Can you work these out from the model? Positions are in its coordinate system, mm. A direction names the side the tool comes from. Round coordinates to 2 decimals unless told otherwise and drop trailing zeros. Write each loop counter-clockwise with the first axis right and the second up, starting at its lowest first coordinate (ties: lowest second). Pieces come first, ordered by that corner, then holes. Notation, with made-up numbers: (13.5, -35) - (35.5, -35) arc R14 cw to (35.5, -19) - close; hole circle Ø4 at (13, 39). An arc over 180 degrees is marked (long way). One line per item, written item: value. Start each with the question number.
(1) I want a section at A-A on z = -2.75. List the corners of the cut face in (x, y) for me.
(2) If I drill on L1, parallel to X at y = 1.3, z = -6; L2, parallel to X at y = 2.2, z = -1.75; L3, parallel to Z at x = 5.5, y = 2.15, over which ranges is the centre line in solid material (lowest first)? Write a range as from..to.
(3) I want a section at D-D on z = 4.75. List the corners of the cut face in (x, y) for me.
(4) I'm going to push flat-ended pins straight in: pin 1 Ø6 at (x, z) = (-21.5, -2.5) entering from -Y; pin 2 Ø1 at (x, y) = (22, 2) entering from -Z; pin 3 Ø0.7 at (x, y) = (2.5, 2) entering from +Z; pin 4 Ø1 at (y, z) = (2, -1) entering from -X. Where does each tip first touch, or does it pass through?
(5) I want a section at C-C on y = 1.05. List the corners of the cut face in (x, z) for me, plus the area to 3 significant figures.
(6) On a 3-axis mill with a long thin cutter (end or side, diameter ignored), from which of +Z, -Z, +X, -X, +Y, -Y can I reach the whole of each face in a straight line? I mean faces 4 (the face through (25.49, 1.89, -5.55)), 5 (the face through (10.699, 0.715, -7.715)), 6 (the face through (0, 2, -6.45)), 7 (the face through (26.35, 2, 0)). Say none if no direction works.
(7) I want a section at B-B on x = -5.5. List the corners of the cut face in (y, z) for me, plus the area to 3 significant figures.
(8) Thinking about a two-plate mould opening in X: for faces 1 (the face through (-28.25, 1, 0)), 2 (the face through (-19, 1, -3)), 3 (the face through (28.25, 1, 0)), which applies, +X half, -X half, draft (parallel to the pull), parting line (faces both ways), or undercut?
from build123d import *

# Parameters (mm, degrees)
BOSS_EXTRUDE1_DEPTH = 1.45
BOSS_EXTRUDE2_DEPTH = 0.9
CUT_EXTRUDE1_DEPTH  = 30.454795874
FILLET1_R           = 1


with BuildPart() as part:
    # Sketch1 → Boss-Extrude1 (new body)
    with BuildSketch(Plane(origin=(0, 0, 0), x_dir=(1, 0, 0), z_dir=(0, 1, 0))):
        with BuildLine():
            Line((-26.25, -8), (26.25, -8))
            ThreePointArc((26.25, -8), (27.664213562, -7.414213562), (28.25, -6))
            Line((28.25, -6), (28.25, 6))
            ThreePointArc((28.25, 6), (27.664213562, 7.414213562), (26.25, 8))
            Line((26.25, 8), (-26.25, 8))
            ThreePointArc((-26.25, 8), (-27.664213562, 7.414213562), (-28.25, 6))
            Line((-28.25, 6), (-28.25, -6))
            ThreePointArc((-28.25, -6), (-27.664213562, -7.414213562), (-26.25, -8))
        make_face()
    extrude(amount=BOSS_EXTRUDE1_DEPTH)

    # Sketch2 → Boss-Extrude2 (add)
    with BuildSketch(Plane(origin=(0, 1.45, 0), x_dir=(1, 0, 0), z_dir=(0, 1, 0))):
        with BuildLine():
            Line((-23.35, -6.45), (23.35, -6.45))
            ThreePointArc((23.35, -6.45), (25.471320344, -5.571320344), (26.35, -3.45))
            Line((26.35, -3.45), (26.35, 3.45))
            ThreePointArc((26.35, 3.45), (25.471320344, 5.571320344), (23.35, 6.45))
            Line((23.35, 6.45), (-23.35, 6.45))
            ThreePointArc((-23.35, 6.45), (-25.471320344, 5.571320344), (-26.35, 3.45))
            Line((-26.35, 3.45), (-26.35, -3.45))
            ThreePointArc((-26.35, -3.45), (-25.471320344, -5.571320344), (-23.35, -6.45))
        make_face()
    extrude(amount=BOSS_EXTRUDE2_DEPTH)

    # Sketch3 → Cut-Extrude1 (cut, through all)
    with BuildSketch(Plane(origin=(0, 2.35, 0), x_dir=(1, 0, 0), z_dir=(0, 1, 0))):
        with BuildLine():
            Line((-19, 0), (-19, 8))
            Line((-19, 8), (-11, 8))
            Line((-11, 8), (-11, 0))
            ThreePointArc((-11, 0), (-15, -4), (-19, 0))
        make_face()
        with BuildLine():
            Line((11, 0), (11, 8))
            Line((11, 8), (19, 8))
            Line((19, 8), (19, 0))
            ThreePointArc((19, 0), (15, -4), (11, 0))
        make_face()
    extrude(amount=-CUT_EXTRUDE1_DEPTH, mode=Mode.SUBTRACT)

    # Fillet1
    fillet1_edges = [part.edges().sort_by_distance(p)[0] for p in [
        (11, 0.725, -8),
        (19, 0.725, -8),
        (-19, 0.725, -8),
        (-11, 0.725, -8),
    ]]
    fillet(fillet1_edges, radius=FILLET1_R)


solid = part.part
Established:
1. outline: (-28.25, 0) - (-19, 0) - (-19, 2.35) - (-26.35, 2.35) - (-26.35, 1.45) - (-28.25, 1.45) - close; (-11, 0) - (11, 0) - (11, 2.35) - (-11, 2.35) - close; (19, 0) - (28.25, 0) - (28.25, 1.45) - (26.35, 1.45) - (26.35, 2.35) - (19, 2.35) - close
2. L1: -28.25..-19, -11..11, 19..28.25
2. L2: -26.35..-19, -11..11, 19..26.35
2. L3: -6.45..6.45
3. outline: (-28.25, 0) - (28.25, 0) - (28.25, 1.45) - (26.05, 1.45) - (26.05, 2.35) - (-26.05, 2.35) - (-26.05, 1.45) - (-28.25, 1.45) - close
4. pin 1: y = 0
4. pin 2: z = -6.45
4. pin 3: z = 6.45
4. pin 4: x = -26.35
5. outline: (-28.25, -6) arc R2 ccw to (-26.25, -8) - (-20, -8) arc R1 ccw to (-19, -7) - (-19, 0) arc R4 cw to (-11, 0) - (-11, -7) arc R1 ccw to (-10, -8) - (10, -8) arc R1 ccw to (11, -7) - (11, 0) arc R4 cw to (19, 0) - (19, -7) arc R1 ccw to (20, -8) - (26.25, -8) arc R2 ccw to (28.25, -6) - (28.25, 6) arc R2 ccw to (26.25, 8) - (-26.25, 8) arc R2 ccw to (-28.25, 6) - close
5. area: 721 mm2
6. face 4: -Z, +X, +Y
6. face 5: -Z, +Y, -Y
6. face 6: -Z, +X, -X, +Y
6. face 7: +Z, -Z, +X, +Y
7. outline: (0, -8) - (1.45, -8) - (1.45, -6.45) - (2.35, -6.45) - (2.35, 6.45) - (1.45, 6.45) - (1.45, 8) - (0, 8) - close
7. area: 34.8 mm2
8. face 1: -X half
8. face 2: undercut
8. face 3: +X half
